Check sheet for the drawn part. Datum: minimum x, y, z corner. Units: mm. Round coordinates to 2 decimals unless told otherwise and drop trailing zeros. Order: outer loops, then holes, each group sorted by start corner. A loop starts at its lowest first (then second) coordinate and runs counter-clockwise, first axis right, second up. Notation, with made-up numbers: (57, -36) -> (78, -36) arc R9 ccw to (78, -24) -> close; hole circle Ø1 at (22.25, -3). An arc over 180 degrees is marked (long way). Answer as CSV lines item,"result". Start each with the question number.
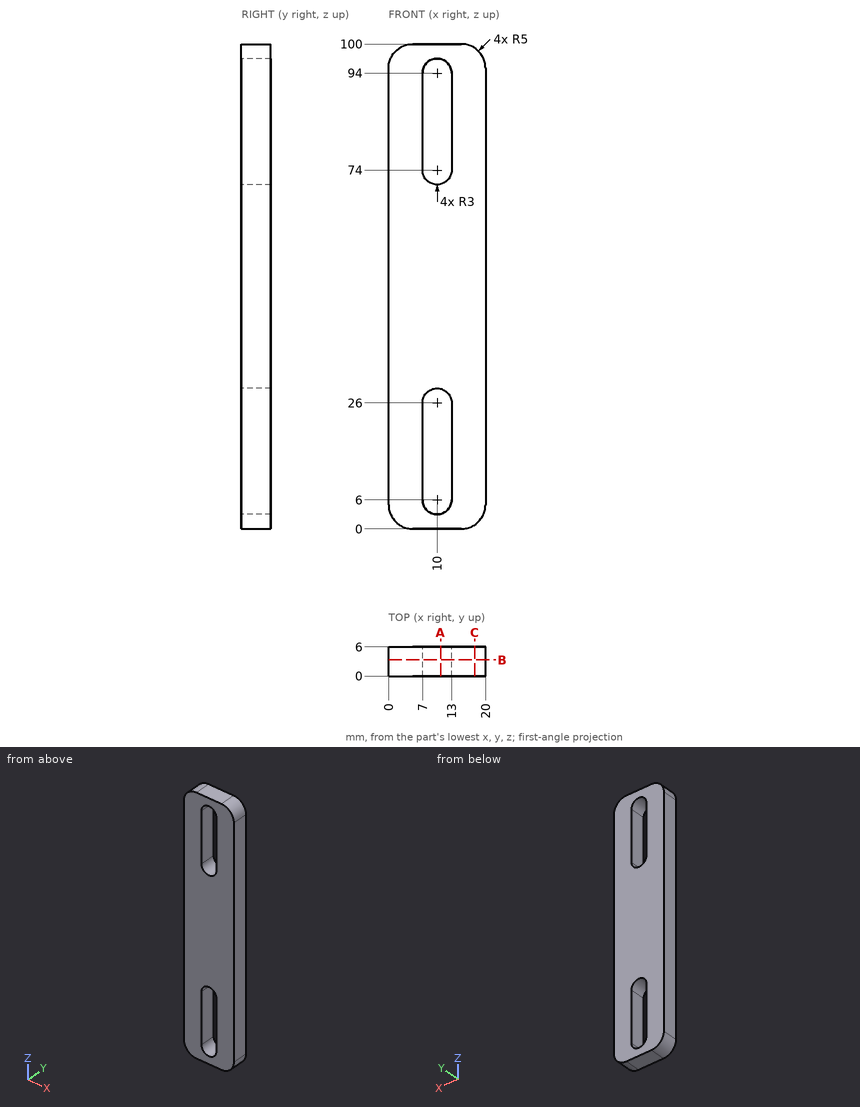
1) Material ranges on line 1 along X through (y, z) = (4.7, 94); line 2 along Z through (x, y) = (9.25, 4.4); line 3 along Z through (x, y) = (10.5, 4.6), recorded low to high.
2) Section check A-A on x = 10.75. Record the cut outline in (y, z), then the cut area to 3 significant figures.
3) Section check B-B on y = 3.3. Record the cut outline in (x, z), then the cut area to 3 significant figures.
4) Section check C-C on x = 17.75. Record the cut outline in (y, z), then the cut area to 3 significant figures.
Solutions:
1,line 1,"x = 0 to 7, 13 to 20"
1,line 2,"z = 0 to 3.1, 28.9 to 71.1, 96.9 to 100"
1,line 3,"z = 0 to 3.04, 28.96 to 71.04, 96.96 to 100"
2,outline,"(0, 0) -> (6, 0) -> (6, 3.1) -> (0, 3.1) -> close; (0, 28.9) -> (6, 28.9) -> (6, 71.1) -> (0, 71.1) -> close; (0, 96.9) -> (6, 96.9) -> (6, 100) -> (0, 100) -> close"
2,area,"290 mm^2"
3,outline,"(0, 5) arc R5 ccw to (5, 0) -> (15, 0) arc R5 ccw to (20, 5) -> (20, 95) arc R5 ccw to (15, 100) -> (5, 100) arc R5 ccw to (0, 95) -> close; hole (7, 6) arc R3 ccw to (13, 6) -> (13, 26) arc R3 ccw to (7, 26) -> close; hole (7, 74) arc R3 ccw to (13, 74) -> (13, 94) arc R3 ccw to (7, 94) -> close"
3,area,"1,680 mm^2"
4,outline,"(0, 0.82) -> (6, 0.82) -> (6, 99.18) -> (0, 99.18) -> close"
4,area,"590 mm^2"
